Part model, mm, in its own coordinate system. Face numbers are marked on the shaded views. A direction names the side the tool comes from. Coordinates: 2 decimals unless noted, no trailing zeros. Loops run counter-clockwise (first coordinate to the right, second up) from the corner with the lowest first, then second, coordinate; pieces in that order, holes last. Notation, with made-up numbers: (71.25, 1.5) - (81.25, 1.5) arc R22 cw to (81.25, 20.5) - close; hole circle Ø5 at (-37.5, 13.25). An arc over 180 degrees is marked (long way). Use a Markdown table: item, result. Add a question column.
1. Pull direction X, two halves, no side cores. Call the marked faces 3, 4 and 5: pulls with the +X half, pulls with the -X half, needs draft (parallel to the pull), parting line crosses it, or undercut.
2. Wall check: probe 1 along Y at (x, z) = (16, -13.5); probe 2 along X at (y, z) = (19.5, -15); probe 3 along X at (y, z) = (19, 5.5). Give the ranges that are in metal, low to high. Write a range as [from, to].
3. 3-axis set-ups, long thin cutter, end or side, ignore diameter. For the marked faces 1 and 2: which of +Z, -Z, +X, -X, +Y, -Y reach the whole face in a straight line?
4. Band-saw the part on B-B, the plane x = 0. Give the cut face in (y, z).
5. Band-saw the part on D-D, the plane x = 20. Give the cut face in (y, z).
6. Band-saw the part on A-A, the plane y = 27. Give the cut face in (x, z).
7. Band-saw the part on C-C, the plane z = -15. Give the cut face in (x, y), plus the area to 3 significant figures.
from build123d import *

# Parameters (mm, degrees)
SKETCH1_W           = 50
SKETCH1_H           = 50
BOSS_EXTRUDE1_DEPTH = 40
SKETCH2_W           = 50
SKETCH2_H           = 50
BOSS_EXTRUDE2_DEPTH = 15
BOSS_EXTRUDE2_TAPER = 30
FILLET1_R           = 3
SHELL1_T            = -2


with BuildPart() as part:
    # Sketch1 → Boss-Extrude1 (new body)
    with BuildSketch(Plane.XY):
        with Locations((5, 32.5)):
            Rectangle(SKETCH1_W, SKETCH1_H)
    extrude(amount=-BOSS_EXTRUDE1_DEPTH)

    # Sketch2 → Boss-Extrude2 (add)
    with BuildSketch(Plane.XY):
        with Locations((5, 32.5)):
            Rectangle(SKETCH2_W, SKETCH2_H)
    extrude(amount=BOSS_EXTRUDE2_DEPTH, taper=BOSS_EXTRUDE2_TAPER)

    # Fillet1
    fillet1_edges = [part.edges().sort_by_distance(p)[0] for p in [
        (30, 7.5, -20),
        (-20, 7.5, -20),
        (-20, 57.5, -20),
        (30, 57.5, -20),
    ]]
    fillet(fillet1_edges, radius=FILLET1_R)

    # Shell1
    shell1_openings = [part.faces().sort_by_distance(p)[0] for p in [
        (5, 32.5, -40),
        (5, 32.5, 15),
    ]]
    offset(amount=SHELL1_T, openings=shell1_openings, kind=Kind.INTERSECTION)


solid = part.part
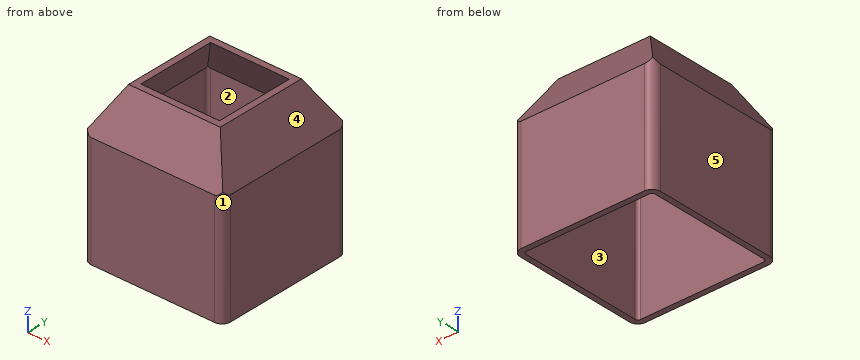
Geometry check:
| question | item | result |
|---|---|---|
| 1 | face 3 | undercut |
| 1 | face 4 | pulls with the +X half |
| 1 | face 5 | pulls with the -X half |
| 2 | probe 1 | y = [7.5, 9.5], [55.5, 57.5] |
| 2 | probe 2 | x = [-20, -18], [28, 30] |
| 2 | probe 3 | x = [-16.82, -14.52], [24.52, 26.82] |
| 3 | face 1 | +Z, -Z, +X, -Y |
| 3 | face 2 | -Z |
| 4 | outline | (7.5, -40) - (9.5, -40) - (9.5, -0.54) - (18.47, 15) - (16.16, 15) - (7.5, 0) - close; (46.53, 15) - (55.5, -0.54) - (55.5, -40) - (57.5, -40) - (57.5, 0) - (48.84, 15) - close |
| 5 | outline | (7.5, -40) - (9.5, -40) - (9.5, -0.54) - (17.5, 13.32) - (47.5, 13.32) - (55.5, -0.54) - (55.5, -40) - (57.5, -40) - (57.5, 0) - (48.84, 15) - (16.16, 15) - (7.5, 0) - close |
| 6 | outline | (-20, -40) - (-18, -40) - (-18, -0.54) - (-9.03, 15) - (-11.34, 15) - (-20, 0) - close; (19.03, 15) - (28, -0.54) - (28, -40) - (30, -40) - (30, 0) - (21.34, 15) - close |
| 7 | outline | (-20, 10.5) arc R3 ccw to (-17, 7.5) - (27, 7.5) arc R3 ccw to (30, 10.5) - (30, 54.5) arc R3 ccw to (27, 57.5) - (-17, 57.5) arc R3 ccw to (-20, 54.5) - close; hole (-18, 10.5) arc R1 ccw to (-17, 9.5) - (27, 9.5) arc R1 ccw to (28, 10.5) - (28, 54.5) arc R1 ccw to (27, 55.5) - (-17, 55.5) arc R1 ccw to (-18, 54.5) - close |
| 7 | area | 377 mm^2 |
